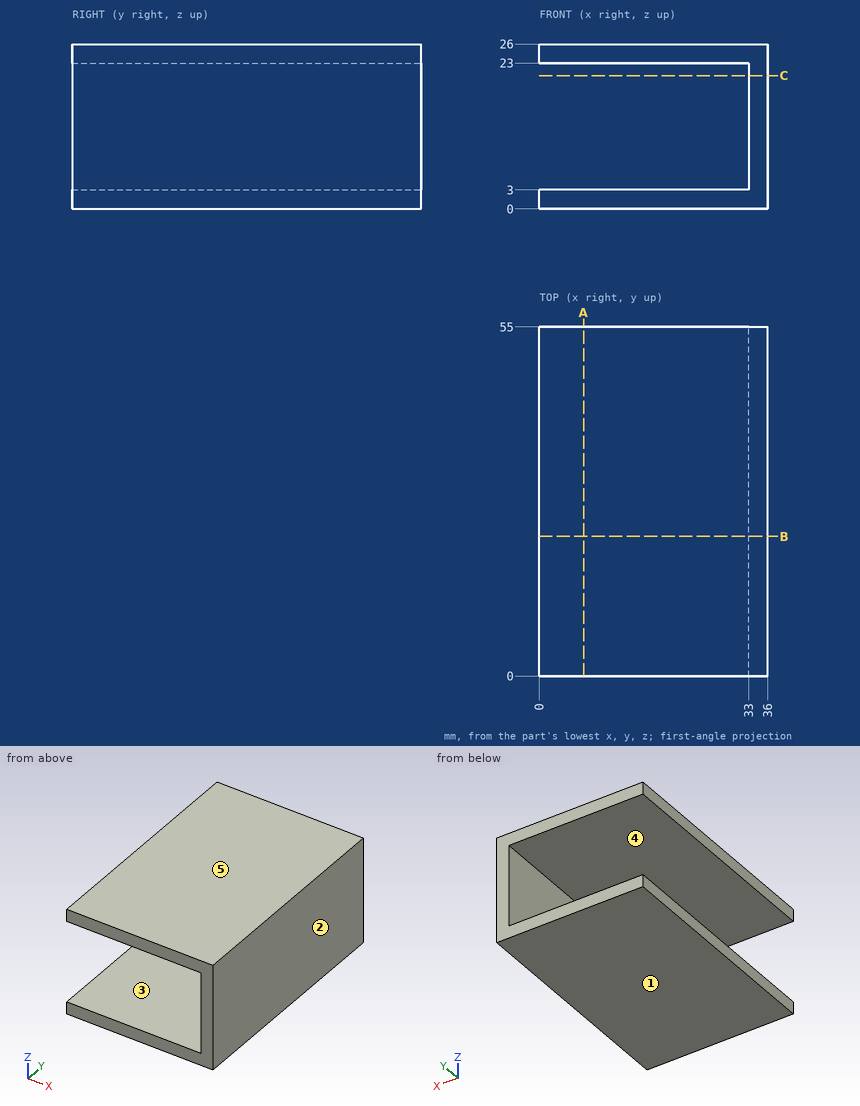
For this review, use the dimensioned drawing (mm, ordinates from the lowest corner) and the shaded views. A direction names the side the tool comes from. Round coordinates to 2 decimals unless told otherwise and drop trailing zeros. Order: outer loops, then holes, each group sorted by start corner. A loop starts at its lowest first (then second) coordinate and runs counter-clockwise, first axis right, second up. Notation, with made-up numbers: (41.25, 85.5) -> (98.25, 85.5) arc R20 cw to (98.25, 97.5) -> close; hole circle Ø7 at (-3, -25). An arc over 180 degrees is marked (long way). Put each result on its own line as item: value.
Q1. Add section A-A on x = 7. Write out the cut boundary in (y, z), plus the area to 3 significant figures.
Check result:
outline: (0, 0) -> (55, 0) -> (55, 3) -> (0, 3) -> close; (0, 23) -> (55, 23) -> (55, 26) -> (0, 26) -> close
area: 330 mm2
Q2. For probe 1 along Z at (x, y) = (22, 37); probe 2 along X at (y, z) = (10, 20.25), list the stretches that pass through material, from the lowest coordinate up. Write a range as [from, to].
Check result:
probe 1: [0, 3], [23, 26]
probe 2: [33, 36]
Q3. Machinability: for the marked faces 4 and 5, which of the approach directions +Z, -Z, +X, -X, +Y, -Y give a long, thin tool a straight path to every point of the face, cutting with its end or side? Answer none if there is none.
Check result:
face 4: -X, +Y, -Y
face 5: +Z, +X, -X, +Y, -Y
Q4. Mouldability with a two-part tool opening along Z and no side actions: class the marked faces 1, 2 and 3 as pulls with the +Z half, pulls with the -Z half, needs draft (parallel to the pull), parting line crosses it, or undercut.
Check result:
face 1: pulls with the -Z half
face 2: needs draft
face 3: undercut
Q5. Add section C-C on z = 21. Write out the cut boundary in (x, y), plus the area to 3 significant figures.
Check result:
outline: (33, 0) -> (36, 0) -> (36, 55) -> (33, 55) -> close
area: 165 mm2
Q6. Insertion check: pin 1 Ø6 at (y, z) = (22.5, 10) entering from -X. The pin has a flat end and moves straight along its axis. Give the tip position at first contact, or say it passes through.
Check result:
pin 1: x = 33
Q7. Add section B-B on y = 22. Write out the cut boundary in (x, z).
Check result:
outline: (0, 0) -> (36, 0) -> (36, 26) -> (0, 26) -> (0, 23) -> (33, 23) -> (33, 3) -> (0, 3) -> close
